Part model, mm, in its own coordinate system. Round coordinates to 2 decimals unless told otherwise and drop trailing zeros. Write each loop counter-clockwise with the first axis right and the second up, starting at its lowest first coordinate (ties: lowest second). Pieces come first, ordered by that corner, then holes. Notation, with made-up numbers: (70, 7.5) -> (117, 7.5) arc R23 ccw to (117, 30.5) -> close; hole circle Ø2 at (64.5, 86.5). An arc over 180 degrees is marked (long way). Return JSON: item names as keys, results as strings. Group by question number.
(1) Saw through at A-A (z = 0.75). List the corners of the cut face in (x, y).
(2) Saw through at B-B (z = -0.5). List the corners of the cut face in (x, y), plus the area to 3 significant figures.
(3) Drop flat-ended pins along their axis: pin 1 Ø3 at (y, z) = (19.5, 1.5) entering from -X; pin 2 Ø0.8 at (x, z) = (20, 5) entering from -Y; pin 3 Ø1.5 at (y, z) = (20.5, -3) entering from -X. Give the stop position or say it passes through.
(4) Mould opens along Y. For faces 1 (the flat face through (20, 19, 6.2)), 2 (the conical face through (19.725, 20.228, -0.35)), 3 (the flat face through (18, 20.3, 6)), 4 (the flat face through (19, 21.1, 5.3)) say: +Y half, -Y half, draft (parallel to the pull), parting line (faces both ways), or undercut.
(5) Drill centre lines: L1, parallel to X at y = 21.4, z = 5; L2, parallel to Y at x = 18.45, z = 2.5; L3, parallel to Z at x = 18.45, y = 17.8. Where is each one in solid material? Low to high. Write a range as from..to.
from build123d import *

# Parameters (mm, degrees)
POCKET001_DEPTH    = 0.3
POLARPATTERN_COUNT = 2
POLARPATTERN_ANGLE = 90


with BuildPart() as part:
    # Sketch013 → Revolution (revolve)
    with BuildSketch(Plane.XZ):
        Polygon((0, 0), (0, -12), (1.5, -1.25), (2.65, -0.1), (2.65, 0), align=None)
    revolve(axis=Axis((0, 0, 0), (0, 0, 1)))

    # Sketch014 → Pocket001 (cut, symmetric)
    with BuildSketch(Plane.XZ):
        Polygon((-2, 0), (0, -2), (2, 0), align=None)
    pocket001 = extrude(amount=POCKET001_DEPTH, both=True, mode=Mode.SUBTRACT)

    # PolarPattern: Pocket001 ×2 about axis
    polarpattern_axis = Axis((0, 0, 0), (0, 0, 1))
    for i in range(1, POLARPATTERN_COUNT):
        add(pocket001.rotate(polarpattern_axis, i * POLARPATTERN_ANGLE / (POLARPATTERN_COUNT - 1)), mode=Mode.SUBTRACT)


with BuildPart() as part_1:
    # Body011 placement: moved
    add(part.part.moved(Location((19, 20, 6.2))))


solid = part_1.part
Computed values:
{
 "1": {"outline": "circle Ø1.83 at (19, 20)"},
 "2": {"outline": "circle Ø1.48 at (19, 20)", "area": "1.72 mm2"},
 "3": {"pin 1": "x = 17.78", "pin 2": "y = 18.28", "pin 3": "x = 18.53"},
 "4": {"face 1": "draft", "face 2": "parting line", "face 3": "undercut", "face 4": "undercut"},
 "5": {"L1": "18.33..19.67", "L2": "18.98..21.02", "L3": "5.72..6.2"}
}
